For this review, take the finished solid that the model builds, in its own axes (mm). A direction names the side the tool comes from. Give positions to 0.01 mm unless a question says otherwise; leave off trailing zeros. Write each loop counter-clockwise with the first axis right and the second up, starting at its lowest first coordinate (ties: lowest second). Pieces come first, ordered by that corner, then holes. Notation, with made-up numbers: M 85,55 L 135,55 A21 ccw 135,74 Z; hole C 17.25,70 d5. An arc over 180 degrees is marked long. Write item = value, one per line.
```python
from build123d import *

# Parameters (mm, degrees)
BOSS_EXTRUDE1_DEPTH      = 17.5
BOSS_EXTRUDE1_DEPTH_BACK = 27.5
SKETCH2_W                = 45
SKETCH2_H                = 4
BOSS_EXTRUDE2_DEPTH      = 15
BOSS_EXTRUDE2_DEPTH_BACK = 15
SKETCH3_R                = 2.5
CUT_EXTRUDE1_DEPTH       = 32.721443851
CUT_EXTRUDE1_DEPTH_BACK  = 32.721443851
RIB1_REACH               = 49.697
SKETCH5_WALL_W           = 111.57136702
SKETCH5_WALL_H           = 5
MIRROR2_COPY_1_REACH     = 49.697
MIRROR2_COPY_1_SKETCH_W  = 111.57136702
MIRROR2_COPY_1_SKETCH_H  = 5
SKETCH7_R                = 2.5
CUT_EXTRUDE2_DEPTH       = 32.721443851
CUT_EXTRUDE2_DEPTH_BACK  = 32.721443851
SKETCH8_R                = 2.875
CUT_EXTRUDE3_DEPTH       = 32.721443851
CUT_EXTRUDE3_DEPTH_BACK  = 32.721443851
SKETCH9_R                = 3.5
CUT_EXTRUDE4_DEPTH       = 15
CUT_EXTRUDE4_DEPTH_BACK  = 32.721443955
SKETCH10_R               = 4
CUT_EXTRUDE5_DEPTH       = 32.721443955
CUT_EXTRUDE5_DEPTH_BACK  = 32.721443955


with BuildPart() as part:
    # Sketch1 → Boss-Extrude1 (new, two sides)
    with BuildSketch(Plane.XY) as boss_extrude1_sk:
        with BuildLine():
            Line((-5, 0), (-5, -5))
            Line((-5, -5), (5, -5))
            Line((5, -5), (5, 0))
            ThreePointArc((5, 0), (0, 5), (-5, 0))
        make_face()
    extrude(amount=BOSS_EXTRUDE1_DEPTH)
    extrude(boss_extrude1_sk.sketch, amount=-BOSS_EXTRUDE1_DEPTH_BACK)

    # Sketch2 → Boss-Extrude2 (add, two sides)
    with BuildSketch(Plane(origin=(0, 0, 0), x_dir=(0, 0, -1), z_dir=(1, 0, 0))) as boss_extrude2_sk:
        with Locations((5, -3)):
            Rectangle(SKETCH2_W, SKETCH2_H)
    extrude(amount=BOSS_EXTRUDE2_DEPTH)
    extrude(boss_extrude2_sk.sketch, amount=-BOSS_EXTRUDE2_DEPTH_BACK)

    # Sketch3 → Cut-Extrude1 (cut, two sides)
    with BuildSketch(Plane.XY) as cut_extrude1_sk:
        Circle(SKETCH3_R)
    extrude(amount=CUT_EXTRUDE1_DEPTH, mode=Mode.SUBTRACT)
    extrude(cut_extrude1_sk.sketch, amount=-CUT_EXTRUDE1_DEPTH_BACK, mode=Mode.SUBTRACT)

    # Sketch5 wall → Rib1 (add, up to next)
    with BuildSketch(Plane(origin=(8.486476183, 1.797142734, 17.5), x_dir=(0.918857093708, -0.394590472949, 0), z_dir=(0.394590472949, 0.918857093708, 0)), mode=Mode.PRIVATE) as rib1_sk1:
        with Locations((0, 2.5)):
            Rectangle(SKETCH5_WALL_W, SKETCH5_WALL_H)
    rib1_tool1 = extrude(rib1_sk1.sketch, amount=-RIB1_REACH, mode=Mode.PRIVATE) - part.part
    rib1 = rib1_tool1.solids().sort_by_distance((8.486476183, 1.797142734, 17.5))[0]
    add(rib1)

    # Mirror1: Rib1 across plane
    add(rib1.mirror(Plane.XY))

    # Mirror2: Rib1 across plane
    add(rib1.mirror(Plane(origin=(0, 0, 0), x_dir=(0, 0, 1), z_dir=(1, 0, 0))))

    # Mirror2 copy 1 sketch → Mirror2 copy 1 (add, up to next)
    with BuildSketch(Plane(origin=(-8.486476183, 1.797142734, -17.5), x_dir=(-0.918857093708, -0.394590472949, 0), z_dir=(-0.394590472949, 0.918857093708, 0)), mode=Mode.PRIVATE) as mirror2_copy_1_sk1:
        with Locations((0, 2.5)):
            Rectangle(MIRROR2_COPY_1_SKETCH_W, MIRROR2_COPY_1_SKETCH_H)
    mirror2_copy_1_tool1 = extrude(mirror2_copy_1_sk1.sketch, amount=-MIRROR2_COPY_1_REACH, mode=Mode.PRIVATE) - part.part
    add(mirror2_copy_1_tool1.solids().sort_by_distance((-8.486476183, 1.797142734, -17.5))[0])

    # Sketch7 → Cut-Extrude2 (cut, two sides)
    with BuildSketch(Plane(origin=(0, 0, 0), x_dir=(1, 0, 0), z_dir=(0, 1, 0))) as cut_extrude2_sk:
        with Locations(Location((-10, 0, 0), (0, 0, 270))):
            Circle(SKETCH7_R)
        with Locations(Location((10, 0, 0), (0, 0, 270))):
            Circle(SKETCH7_R)
    extrude(amount=CUT_EXTRUDE2_DEPTH, mode=Mode.SUBTRACT)
    extrude(cut_extrude2_sk.sketch, amount=-CUT_EXTRUDE2_DEPTH_BACK, mode=Mode.SUBTRACT)

    # Sketch8 → Cut-Extrude3 (cut, two sides)
    with BuildSketch(Plane(origin=(0, 0, 0), x_dir=(1, 0, 0), z_dir=(0, 1, 0))) as cut_extrude3_sk:
        with Locations(Location((0, 12.5, 0), (0, 0, 46.666459534))):
            Circle(SKETCH8_R)
    extrude(amount=CUT_EXTRUDE3_DEPTH, mode=Mode.SUBTRACT)
    extrude(cut_extrude3_sk.sketch, amount=-CUT_EXTRUDE3_DEPTH_BACK, mode=Mode.SUBTRACT)

    # Sketch9 → Cut-Extrude4 (cut, two sides)
    with BuildSketch(Plane.XY) as cut_extrude4_sk:
        Circle(SKETCH9_R)
    extrude(amount=CUT_EXTRUDE4_DEPTH, mode=Mode.SUBTRACT)
    extrude(cut_extrude4_sk.sketch, amount=-CUT_EXTRUDE4_DEPTH_BACK, mode=Mode.SUBTRACT)

    # Sketch10 → Cut-Extrude5 (cut, two sides)
    with BuildSketch(Plane(origin=(0, 0, 0), x_dir=(1, 0, 0), z_dir=(0, 1, 0))) as cut_extrude5_sk:
        with Locations(Location((0, 22, 0), (0, 0, 90))):
            Circle(SKETCH10_R)
    extrude(amount=CUT_EXTRUDE5_DEPTH, mode=Mode.SUBTRACT)
    extrude(cut_extrude5_sk.sketch, amount=-CUT_EXTRUDE5_DEPTH_BACK, mode=Mode.SUBTRACT)


solid = part.part
```
1. Machinability: for faces 5 (the face through (-8, 1, 12.5)), 6 (the face through (8, 1, 12.5)), 7 (the face through (-5, -0.5, -22.4)), 8 (the face through (2, -2, 15)), 9 (the face through (7.56, -2.97, -0.54)), which of the approach directions +Z, -Z, +X, -X, +Y, -Y give a long, thin tool a straight path to every point of the face, cutting with its end or side? Answer none if there is none.
Responses:
face_5 = -X, +Y
face_6 = +X, +Y
face_7 = -Z, -X, +Y
face_8 = -Z
face_9 = +Y, -Y
2. For line 1 along X through (y, z) = (-4.1, -12.5) (3 decimals); line 2 along X through (y, z) = (-2.2, -22); line 3 along Y through (x, z) = (0, 17.05), list the stretches that pass through material, from the lowest coordinate up. Write a range as from..to.
Responses:
line_1 = -15..-2.875, 2.875..15
line_2 = -15..-4, 4..15
line_3 = -5..-2.5, 2.5..5
3. We need section D-D, the plane y = 1. Write out the cut boundary in (x, z).
Responses:
outline = M -10.34,-17.5 L -4.9,-17.5 L -4.9,-27.5 L -3.35,-27.5 L -3.35,-24.18 A4 cw -3.35,-19.82 L -3.35,15 L -2.29,15 L -2.29,17.5 L -10.34,17.5 L -10.34,12.5 L -4.9,12.5 L -4.9,-12.5 L -10.34,-12.5 Z; M 2.29,15 L 3.35,15 L 3.35,-19.82 A4 cw 3.35,-24.18 L 3.35,-27.5 L 4.9,-27.5 L 4.9,-17.5 L 10.34,-17.5 L 10.34,-12.5 L 4.9,-12.5 L 4.9,12.5 L 10.34,12.5 L 10.34,17.5 L 2.29,17.5 Z
4. The part is to be moulded in two halves that separate along Y. For faces 1 (the face through (-8.395, 1.836, 14.965)), 2 (the face through (0, -5, -5)), 3 (the face through (-12.44, -2.97, -0.54)), 4 (the face through (-0.759, -3.417, -26.089)), say which applies: +Y half, -Y half, draft (parallel to the pull), parting line (faces both ways), or undercut.
Responses:
face_1 = +Y half
face_2 = -Y half
face_3 = draft
face_4 = undercut
5. We need section C-C, the plane z = -4. Write out the cut boundary in (x, y), then the cut area to 3 significant figures.
Responses:
outline = M -15,-5 L 15,-5 L 15,-1 L 5,-1 L 5,0 A5 ccw -5,0 L -5,-1 L -15,-1 Z; hole C 0,0 d7
area = 131 mm2
6. Insertion check: P1, Ø2, axis at x = -0.5, z = -3, coming from the +Y side; P2, Ø3.5, axis at x = -1.5, y = 0.5, coming from the -Z side; P3, Ø5, axis at x = 9, z = 6, coming from the +Y side; P4, Ø6, axis at x = 8.5, y = 2.5, coming from the -Z side. Each pin has a flat end and moves straight along its axis. Give the tip position at first contact, or say it passes through.
Responses:
P1 = 5
P2 = 15
P3 = -1
P4 = -17.5
7. We need section B-B, the plane x = 0. Write out the cut boundary in (y, z) (3 decimals), then the cut area to 4 significant figures.
Responses:
outline = M -5,-27.5 L -3.5,-27.5 L -3.5,-26 L -5,-26 Z; M -5,-18 L -3.5,-18 L -3.5,-15.375 L -5,-15.375 Z; M -5,-9.625 L -3.5,-9.625 L -3.5,15 L -2.5,15 L -2.5,17.5 L -5,17.5 Z; M 2.5,15 L 3.5,15 L 3.5,-9.625 L 5,-9.625 L 5,17.5 L 2.5,17.5 Z; M 3.5,-27.5 L 5,-27.5 L 5,-26 L 3.5,-26 Z; M 3.5,-18 L 5,-18 L 5,-15.375 L 3.5,-15.375 Z
area = 98.75 mm2
8. We need section A-A, the plane z = 2. Write out the cut boundary in (x, y), then the cut area to 3 significant figures.
Responses:
outline = M -15,-5 L -11.5,-5 L -11.5,-1 L -15,-1 Z; M -8.5,-5 L 8.5,-5 L 8.5,-1 L 5,-1 L 5,0 A5 ccw -5,0 L -5,-1 L -8.5,-1 Z; M 11.5,-5 L 15,-5 L 15,-1 L 11.5,-1 Z; hole C 0,0 d7
area = 107 mm2
